Geometry check sheet. Reference: the model listing, model coordinates, mm. Face numbers are marked on the shaded views. Round coordinates to 2 decimals unless told otherwise and drop trailing zeros. Order: outer loops, then holes, each group sorted by start corner. A loop starts at its lowest first (then second) coordinate and runs counter-clockwise, first axis right, second up. Notation, with made-up numbers: (0, 58.25) -> (12, 58.25) arc R9 ccw to (12, 63.25) -> close; hole circle Ø8 at (46.5, 25). An arc over 180 degrees is marked (long way). Answer as a JSON object with one key per item and string values. Group by question number.
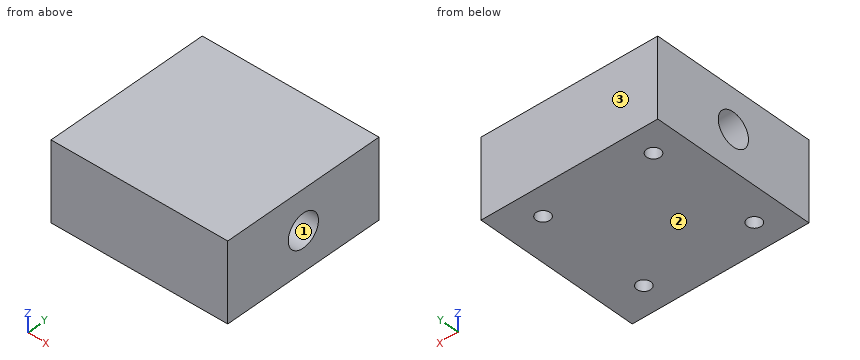
from build123d import *

# Parameters (mm, degrees)
SKETCH1_W                 = 32
SKETCH1_H                 = 30
BOSS_EXTRUDE1_DEPTH       = 7.125
M3X0_5_TAPPED_HOLE1_D     = 2.5
M3X0_5_TAPPED_HOLE1_DEPTH = 7.5
M3X0_5_TAPPED_HOLE1_TIP   = 0.751075774
M6X1_0_TAPPED_HOLE1_D     = 6


with BuildPart() as part:
    # Sketch1 → Boss-Extrude1 (new, symmetric)
    with BuildSketch(Plane.XY):
        Rectangle(SKETCH1_W, SKETCH1_H)
    extrude(amount=BOSS_EXTRUDE1_DEPTH, both=True)

    # M3x0.5 Tapped Hole1
    with Locations(Plane(origin=(0, 0, -7.125), x_dir=(-1, 0, 0), z_dir=(0, 0, -1))):
        with Locations((-9.333333333, 10), (10.666666667, 10), (10.666666667, -10), (-9.333333333, -10)):
            Hole(M3X0_5_TAPPED_HOLE1_D / 2, depth=M3X0_5_TAPPED_HOLE1_DEPTH)
            with Locations((0, 0, -(M3X0_5_TAPPED_HOLE1_DEPTH + M3X0_5_TAPPED_HOLE1_TIP / 2))):  # 118° drill point
                Cone(0, M3X0_5_TAPPED_HOLE1_D / 2, M3X0_5_TAPPED_HOLE1_TIP, mode=Mode.SUBTRACT)

    # M6x1.0 Tapped Hole1 (through all)
    with Locations(Plane(origin=(16, 0, 0), x_dir=(0, 0, -1), z_dir=(1, 0, 0))):
        with Locations((0, 0)):
            Hole(M6X1_0_TAPPED_HOLE1_D / 2)


solid = part.part
Item 1: Sectioned sample at A-A, the plane z = 0. Enter the section's corners in (x, y).
Item 2: Sectioned sample at B-B, the plane y = 0. Enter the section's corners in (x, z) (3 decimals).
Item 3: Depth check by flat-ended pin: pin 1 Ø3 at (x, y) = (-10.67, -10) entering from -Z (3 decimals); pin 2 Ø2 at (x, y) = (9.33, -10) entering from -Z. Enter the tip coordinate at first touch or a pass-through.
Item 4: Sectioned sample at D-D, the plane x = -13. Enter the section's corners in (y, z) (3 decimals), then the cut area to 3 significant figures.
Item 5: Sectioned sample at C-C, the plane z = -4.5. Enter the section's corners in (x, y), then the cut area to 3 significant figures.
Item 6: Mould release check, pull along Z, two halves, no side actions. Record for the marked faces 1, 2 and 3: pulls with the +Z half, pulls with the -Z half, needs draft (parallel to the pull), parting line crosses it, or undercut.
Item 7: Thickness scan on L1, parallel to X at y = 10, z = -4.5; L2, parallel to Y at x = -9, z = 0; L3, parallel to Y at x = 3.5, z = 1. Record the ranges inside material, lowest first.
Result:
{
 "1": {"outline": "(-16, -15) -> (16, -15) -> (16, -3) -> (-16, -3) -> close; (-16, 3) -> (16, 3) -> (16, 15) -> (-16, 15) -> close; hole circle Ø2.5 at (-10.67, -10); hole circle Ø2.5 at (-10.67, 10); hole circle Ø2.5 at (9.33, -10); hole circle Ø2.5 at (9.33, 10)"},
 "2": {"outline": "(-16, -7.125) -> (16, -7.125) -> (16, -3) -> (-16, -3) -> close; (-16, 3) -> (16, 3) -> (16, 7.125) -> (-16, 7.125) -> close"},
 "3": {"pin 1": "stops at z = -7.125", "pin 2": "stops at z = 0.52"},
 "4": {"outline": "(-15, -7.125) -> (15, -7.125) -> (15, 7.125) -> (-15, 7.125) -> close; hole circle Ø6 at (0, 0)", "area": "399 mm2"},
 "5": {"outline": "(-16, -15) -> (16, -15) -> (16, 15) -> (-16, 15) -> close; hole circle Ø2.5 at (-10.67, -10); hole circle Ø2.5 at (-10.67, 10); hole circle Ø2.5 at (9.33, -10); hole circle Ø2.5 at (9.33, 10)", "area": "940 mm2"},
 "6": {"face 1": "undercut", "face 2": "pulls with the -Z half", "face 3": "needs draft"},
 "7": {"L1": "x = -16 to -11.92, -9.42 to 8.08, 10.58 to 16", "L2": "y = -15 to -3, 3 to 15", "L3": "y = -15 to -2.83, 2.83 to 15"}
}
